Autodesk Inventor part; units mm, degrees
ref_plane "YZ Plane" through (0, 0, 0) normal (1, 0, 0) x (0, 1, 0)
ref_plane "XZ Plane" through (0, 0, 0) normal (0, 1, 0) x (-1, 0, 0)
ref_plane "XY Plane" through (0, 0, 0) normal (0, 0, 1) x (1, 0, 0)
sketch "Sketch1" plane through (0, 0, 0) normal (0, 0, 1) x (1, 0, 0)
  line L0 (-14.0074, 10.2243) -> (11.3926, 10.2243)
  line L1 (11.3926, 10.2243) -> (11.3926, -15.1757)
  line L2 (11.3926, -15.1757) -> (-14.0074, -15.1757)
  line L3 (-14.0074, -15.1757) -> (-14.0074, 10.2243)
  line L4 (10.1226, 8.9543) -> (-12.7374, 8.9543)
  line L5 (-12.7374, 8.9543) -> (-12.7374, -13.9057)
  line L6 (-12.7374, -13.9057) -> (10.1226, -13.9057)
  line L7 (10.1226, -13.9057) -> (10.1226, 8.9543)
  point P0 (0, 0)
  dimension "d0" = 25.4
  dimension "d1" = 1.27
extrude "Extrusion2" add sketch "Sketch1" along normal blind 660.4
equation "\"d4\" = d2"
equation "\"d2\" = 660.4"
properties part number "1x1 Stock 26in"
Read the model definition and answer for the solid it produces. Units are mm, in the model's axes. A direction names the side the tool comes from. Coordinates: 2 decimals unless noted, no trailing zeros. Loops run counter-clockwise (first coordinate to the right, second up) from the corner with the lowest first, then second, coordinate; pieces in that order, holes last. Notation, with made-up numbers: (51, 82.25) - (76, 82.25) arc R10 cw to (76, 88.25) - close; hole circle Ø4 at (75, 89). An arc over 180 degrees is marked (long way). Answer in a Markdown table with one row per item.
Q1. Find section A-A on y = -7.75. Write down the section's boundary in (x, z), plus the area to 3 significant figures.
Here are the results:
| item | result |
|---|---|
| outline | (-14.01, 0) - (-12.74, 0) - (-12.74, 660.4) - (-14.01, 660.4) - close; (10.12, 0) - (11.39, 0) - (11.39, 660.4) - (10.12, 660.4) - close |
| area | 1,680 mm^2 |
Q2. Given P1, Ø6, axis at x = -7, y = 3, coming from the -Z side, flat-ended and moving along its own axis, determine where the tip first touches the part or whether it passes through.
Here are the results:
| item | result |
|---|---|
| P1 | passes through |
Q3. Find section C-C on z = 156. Write down the section's boundary in (x, y).
Here are the results:
| item | result |
|---|---|
| outline | (-14.01, -15.18) - (11.39, -15.18) - (11.39, 10.22) - (-14.01, 10.22) - close; hole (-12.74, -13.91) - (10.12, -13.91) - (10.12, 8.95) - (-12.74, 8.95) - close |
Q4. Straight lines are drawn through the part: line 1 along X through (y, z) = (-2.75, 166.5); line 2 along Y through (x, z) = (6.25, 555). For each, find the intervals that lie inside material, in ascending order. Write a range as [from, to].
Here are the results:
| item | result |
|---|---|
| line 1 | x = [-14.01, -12.74], [10.12, 11.39] |
| line 2 | y = [-15.18, -13.91], [8.95, 10.22] |
Q5. The mould has two halves that part along Y. Classify faces 1 (the flat face through (-1, -13.906, 326)), 2 (the flat face through (-2, -15, 660.4)), 3 (the flat face through (-1, 10.224, 326)): pulls with the +Y half, pulls with the -Y half, needs draft (parallel to the pull), parting line crosses it, or undercut.
Here are the results:
| item | result |
|---|---|
| face 1 | undercut |
| face 2 | needs draft |
| face 3 | pulls with the +Y half |
Q6. For faces 4 (the flat face through (-12.737, -2, 326)), 5 (the flat face through (11.393, -2, 326)), determine the directions among +Z, -Z, +X, -X, +Y, -Y from which every point of the face is accessible in a straight line to the end or side of a thin tool.
Here are the results:
| item | result |
|---|---|
| face 4 | +Z, -Z |
| face 5 | +Z, -Z, +X, +Y, -Y |
Q7. Find section B-B on x = -6.5. Write down the section's boundary in (y, z), plus the area to 3 significant figures.
Here are the results:
| item | result |
|---|---|
| outline | (-15.18, 0) - (-13.91, 0) - (-13.91, 660.4) - (-15.18, 660.4) - close; (8.95, 0) - (10.22, 0) - (10.22, 660.4) - (8.95, 660.4) - close |
| area | 1,680 mm^2 |
